Could you check a few things on this model? Use its own coordinates, in mm. Face numbers are marked on the shaded views. A direction names the side the tool comes from. Give positions to 0.01 mm unless a question says otherwise; leave off trailing zeros. Write each loop counter-clockwise with the first axis right and the second up, starting at its lowest first coordinate (ties: lowest second). Pieces come first, ordered by that corner, then holes. Notation, with made-up numbers: M 21.25,-25.75 L 36.25,-25.75 A6 cw 36.25,-16.75 Z; hole C 12.5,33.25 d11. An arc over 180 degrees is marked long. Answer as CSV lines item,"result". Start each with the question number.
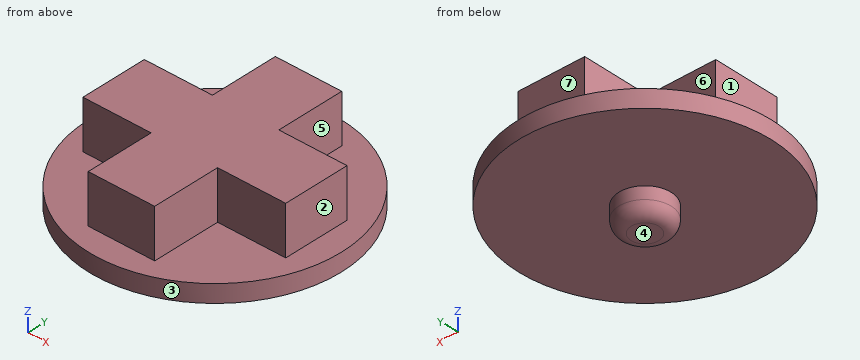
from build123d import *

# Parameters (mm, degrees)
SKETCH1_R           = 12.85
BOSS_EXTRUDE1_DEPTH = 1.8
BOSS_EXTRUDE2_DEPTH = 4.95
SKETCH3_R           = 2.65
BOSS_EXTRUDE3_DEPTH = 2.5
FILLET1_R           = 1.25


with BuildPart() as part:
    # Sketch1 → Boss-Extrude1 (new body)
    with BuildSketch(Plane.XY):
        Circle(SKETCH1_R)
    extrude(amount=BOSS_EXTRUDE1_DEPTH)

    # Sketch2 → Boss-Extrude2 (add)
    with BuildSketch(Plane.XY.offset(1.8)):
        Polygon((3.375, 3.375), (10.3, 3.375), (10.3, -3.375), (3.375, -3.375), (3.375, -10.3), (-3.375, -10.3), (-3.375, -3.375), (-10.3, -3.375), (-10.3, 3.375), (-3.375, 3.375), (-3.375, 10.3), (3.375, 10.3), align=None)
    extrude(amount=BOSS_EXTRUDE2_DEPTH)

    # Sketch3 → Boss-Extrude3 (add)
    with BuildSketch(Plane(origin=(0, 0, 0), x_dir=(-1, 0, 0), z_dir=(0, 0, -1))):
        with Locations(Location((0, 0, 0), (0, 0, 180))):
            Circle(SKETCH3_R)
    extrude(amount=BOSS_EXTRUDE3_DEPTH)

    # Fillet1
    fillet1_edges = [part.edges().sort_by_distance(p)[0] for p in [
        (-2.65, 0, -2.5),
    ]]
    fillet(fillet1_edges, radius=FILLET1_R)


solid = part.part
1. Imagine slicing it at B-B, the plane z = 5.25. Please give me the cut outline in (x, y) (3 decimals).
2. Imagine slicing it at A-A, the plane x = 0. Please give me the cut outline in (y, z), plus the area to 3 significant figures.
3. Will these pins go through, and if not, where does the flat tip stop? P1, Ø1.5, axis at y = -0.5, z = 3, coming from the +X side; P2, Ø4, axis at x = -8.5, z = 3.5, coming from the -Y side; P3, Ø1.5, axis at x = -0.5, z = 5.5, coming from the +Y side.
4. Please list where these lines run through material, in increasing order: line 1 (X direction, y = 7.25, z = 3.25) (3 decimals); line 2 (X direction, y = -2.75, z = 2.75); line 3 (Z direction, x = -5.25, y = -6.25).
5. On a 3-axis mill with a long thin cutter (end or side, diameter ignored), from which of +Z, -Z, +X, -X, +Y, -Y can I reach the whole of each face in a straight line? I mean the marked faces 5, 6 and 7. Say none if no direction works.
6. Imagine slicing it at D-D, the plane y = 8.5. Please give me the cut outline in (x, z) (3 decimals), plus the area to 3 significant figures.
7. Thinking about a two-plate mould opening in X: for the marked faces 1, 2, 3 and 4, which applies, pulls with the +X half, pulls with the -X half, needs draft (parallel to the pull), parting line crosses it, or undercut?
Solutions:
1,outline,"M -10.3,-3.375 L -3.375,-3.375 L -3.375,-10.3 L 3.375,-10.3 L 3.375,-3.375 L 10.3,-3.375 L 10.3,3.375 L 3.375,3.375 L 3.375,10.3 L -3.375,10.3 L -3.375,3.375 L -10.3,3.375 Z"
2,outline,"M -12.85,0 L -2.65,0 L -2.65,-1.25 A1.25 ccw -1.4,-2.5 L 1.4,-2.5 A1.25 ccw 2.65,-1.25 L 2.65,0 L 12.85,0 L 12.85,1.8 L 10.3,1.8 L 10.3,6.75 L -10.3,6.75 L -10.3,1.8 L -12.85,1.8 Z"
2,area,"161 mm²"
3,P1,"x = 10.3"
3,P2,"y = -10.47"
3,P3,"y = 10.3"
4,line 1,"-3.375 to 3.375"
4,line 2,"-10.3 to 10.3"
4,line 3,"0 to 1.8"
5,face 5,"+Z, +X, +Y"
5,face 6,"+Z, -X, +Y"
5,face 7,"+Z, +X, -X, +Y"
6,outline,"M -9.637,0 L 9.637,0 L 9.637,1.8 L 3.375,1.8 L 3.375,6.75 L -3.375,6.75 L -3.375,1.8 L -9.637,1.8 Z"
6,area,"68.1 mm²"
7,face 1,"pulls with the -X half"
7,face 2,"pulls with the +X half"
7,face 3,"parting line crosses it"
7,face 4,"needs draft"
